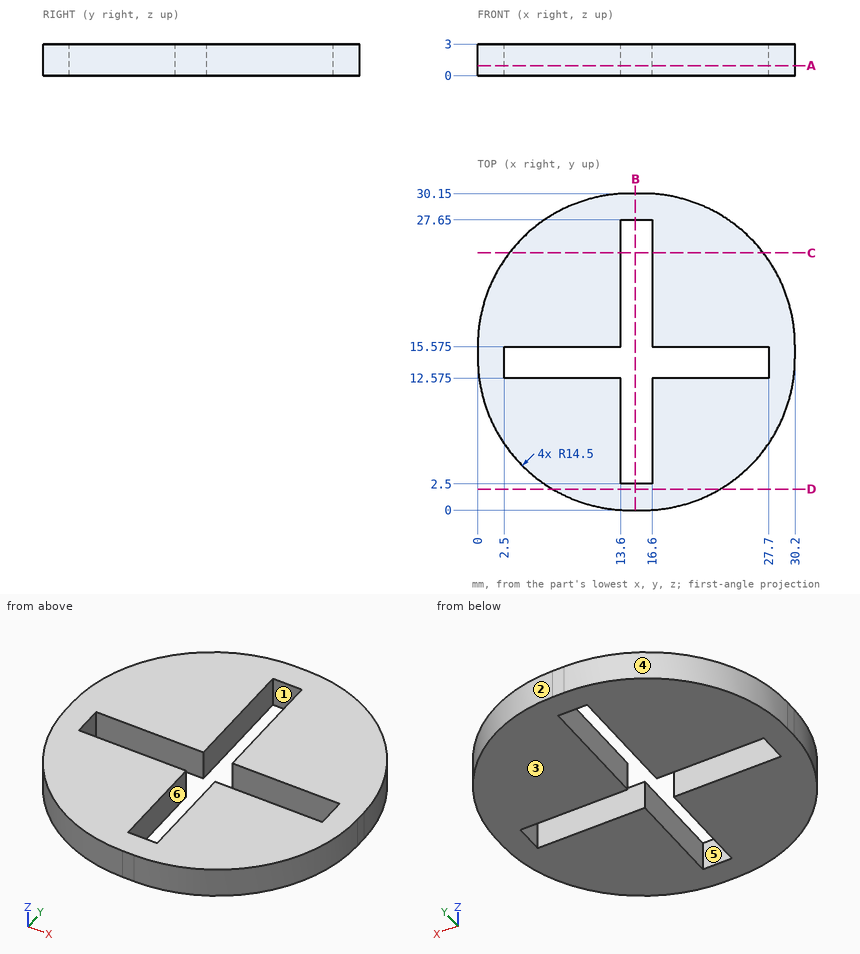
Study the drawing (mm; zero at the part's minimum x, y, z) and answer. A direction names the side the tool comes from. Coordinates: 2 decimals unless noted, no trailing zeros. Write each loop counter-clockwise with the first axis right and the second up, starting at its lowest first coordinate (ties: lowest second). Pieces come first, ordered by that corner, then holes.
Q1. The mould has two halves that part along X. Classify the marked faces 3, 4, 5 and 6: released by +X, released by -X, zero draft, split by the parting line, or undercut.
Returned:
face 3: zero draft
face 4: released by -X
face 5: undercut
face 6: undercut
Q2. Which of the six approach directions +Z, -Z, +X, -X, +Y, -Y give full straight-line access (tool end or side, diameter ignored) to the marked faces 1 and 2?
Returned:
face 1: +Z, -Z
face 2: +Z, -Z, +X, +Y
Q3. Given P1, Ø1.5, axis at y = 23.5, z = 1, coming from the -X side; P2, Ø1, axis at x = 17.5, z = 1, coming from the -Y side; P3, Ø1.5, axis at x = 25, z = 1, coming from the -Y side, each flat-ended and moving along its own axis, determine where each tip first touches the part or whether it passes through.
Returned:
P1: stops at x = 1.86
P2: stops at y = 0.06
P3: stops at y = 2.79
Q4. Find the intervals of material crossed by line 1 along X through (y, z) = (16, 0.9); line 2 along X through (y, z) = (15.5, 0.3); line 3 along Y through (x, z) = (27, 1.3) (3 decimals), in increasing order.
Returned:
line 1: x = 0 to 13.6, 16.6 to 30.2
line 2: x = 0 to 2.5, 27.7 to 30.2
line 3: y = 5.414 to 12.575, 15.575 to 24.736
Q5. Section A-A, the plane z = 0.95 is taken. Write down the section's boundary in (x, y) (3 decimals).
Returned:
outline: (0, 14.5) arc R14.5 ccw to (14.5, 0) - (15.7, 0) arc R14.5 ccw to (30.2, 14.5) - (30.2, 15.65) arc R14.5 ccw to (15.7, 30.15) - (14.5, 30.15) arc R14.5 ccw to (0, 15.65) - close; hole (2.5, 12.575) - (13.6, 12.575) - (13.6, 2.5) - (16.6, 2.5) - (16.6, 12.575) - (27.7, 12.575) - (27.7, 15.575) - (16.6, 15.575) - (16.6, 27.65) - (13.6, 27.65) - (13.6, 15.575) - (2.5, 15.575) - close
Q6. Section D-D, the plane y = 2 is taken. Write down the section's boundary in (x, z).
Returned:
outline: (7.15, 0) - (23.05, 0) - (23.05, 3) - (7.15, 3) - close
Q7. Section B-B, the plane x = 15 is taken. Write down the section's boundary in (y, z), then the cut area to 3 significant figures.
Returned:
outline: (0, 0) - (2.5, 0) - (2.5, 3) - (0, 3) - close; (27.65, 0) - (30.15, 0) - (30.15, 3) - (27.65, 3) - close
area: 15.0 mm2
Q8. Section C-C, the plane y = 24.5 is taken. Write down the section's boundary in (x, z), then the cut area to 3 significant figures.
Returned:
outline: (3.01, 0) - (13.6, 0) - (13.6, 3) - (3.01, 3) - close; (16.6, 0) - (27.19, 0) - (27.19, 3) - (16.6, 3) - close
area: 63.5 mm2
